Autodesk Inventor part; units mm, degrees
ref_plane "YZ Plane" through (0, 0, 0) normal (1, 0, 0) x (0, 1, 0)
ref_plane "XZ Plane" through (0, 0, 0) normal (0, 1, 0) x (-1, 0, 0)
ref_plane "XY Plane" through (0, 0, 0) normal (0, 0, 1) x (1, 0, 0)
sketch "Sketch1" plane through (0, 0, 0) normal (1, 0, 0) x (0, 1, 0)
  circle A0 centre (0, 0) radius 27.051
  dimension "d0" = 54.102
extrude "Extrusion1" add sketch "Sketch1" along normal blind 36.576
sketch "Sketch2" plane through (36.576, 0, 0) normal (1, 0, 0) x (0, 0, -1)
  circle A0 centre (0, 0) radius 6.35
  dimension "d3" = 12.7
extrude "Extrusion2" cut sketch "Sketch2" against normal through all
sketch "Sketch3" plane through (36.576, 0, 0) normal (1, 0, 0) x (0, 0, -1)
  circle A0 centre (0, 0) radius 6.35
  circle A1 centre (0, 0) radius 27.051
  line L0 (0, 0) -> (-36.068, 0) construction
  line L1 (-18.288, -6.0325) -> (-36.068, -6.0325)
  line L2 (-36.068, -6.0325) -> (-36.068, 6.0325)
  line L3 (-36.068, 6.0325) -> (-18.288, 6.0325)
  line L4 (-18.288, 6.0325) -> (-18.288, -6.0325)
  line L5 (-18.288, -6.0325) -> (-36.068, 6.0325) construction
  line L6 (-36.068, -6.0325) -> (-18.288, 6.0325) construction
  circle A2 centre (-30.734, 0) radius 2.921
  line L7 (-30.734, 2.921) -> (-36.068, 2.921)
  line L8 (-30.734, -2.921) -> (-36.068, -2.921)
  point P0 (-27.178, 0)
  dimension "d6" = 27.178
  dimension "d7" = 12.065
  dimension "d8" = 17.78
  dimension "d9" = 5.842
  dimension "d10" = 5.334
extrude "Extrusion3" add sketch "Sketch3" along normal blind 1.524 contours L3 L4 L1 A1 | A1 L1 L2 L8 A2 L7 L3 picked at (-21.1837, 0.6753)
properties part number "SlipRing"
Source: CAD feature listing. Evaluate the final solid. Frame: model axes, mm. A direction names the side the tool comes from. Coordinates: 2 decimals unless noted, no trailing zeros. Loops run counter-clockwise (first coordinate to the right, second up) from the corner with the lowest first, then second, coordinate; pieces in that order, holes last. Notation, with made-up numbers: (19, -11) - (75, -11) arc R7 cw to (75, -2) - close; hole circle Ø6 at (-35, -18). An arc over 180 degrees is marked (long way). One line per question, with ' | ' between items.
1) Pull-direction query (Y, two-part tool) for faces 4 (the face through (37, 2.921, 33)), 5 (the face through (37, -6.032, 27)), 6 (the face through (37, 6.032, 27)), 7 (the face through (18.54, -6.2, 1.38)); classes: released by +Y, released by -Y, zero draft, split by the parting line, or undercut.
Report:
face 4: undercut | face 5: released by -Y | face 6: released by +Y | face 7: undercut
2) Section C-C, the plane x = 21.5. Return loops of the section in (y, z).
Report:
outline: circle Ø54.1 at (0, 0); hole circle Ø12.7 at (0, 0)
3) First-contact query: P1, Ø2, axis at x = 27.5, z = 9, coming from the +Y side; P2, Ø1.5, axis at x = 10, z = 6, coming from the -Y side; P3, Ø10.5, axis at y = 0, z = 33.5, coming from the -X side. Flat tips, straight axial feed; report the tip coordinate or a pass-through.
Report:
P1: stops at y = 25.84 | P2: stops at y = -26.54 | P3: stops at x = 36.58
4) Set-up query: faces 1 (the face through (38.1, 0, 25)), 2 (the face through (37, -2.921, 33)), 3 (the face through (37, 0, 18.288)). Return all of +Z, -Z, +X, -X, +Y, -Y with unobstructed straight access to the full face (end or side cutting, diameter ignored); none if empty.
Report:
face 1: +Z, -Z, +X, +Y, -Y | face 2: +Z, +X, -X | face 3: -Z, +X, +Y, -Y
5) Section B-B, the plane z = 0. Return loops of the section in (x, y), then the cut area to 3 significant figures.
Report:
outline: (0, -27.05) - (36.58, -27.05) - (36.58, -6.35) - (0, -6.35) - close; (0, 6.35) - (36.58, 6.35) - (36.58, 27.05) - (0, 27.05) - close | area: 1,510 mm²
6) Section D-D, the plane y = 10. Return loops of the section in (x, z), then the cut area to 3 significant figures.
Report:
outline: (0, -25.13) - (36.58, -25.13) - (36.58, 25.13) - (0, 25.13) - close | area: 1,840 mm²
7) Line query: line 1 along Y through (x, z) = (27, 0); line 2 along X through (y, z) = (-15.5, 12.5); line 3 along Y through (x, z) = (6.5, -4). Output: solid intervals per line, ascending.
Report:
line 1: y = -27.05 to -6.35, 6.35 to 27.05 | line 2: x = 0 to 36.58 | line 3: y = -26.75 to -4.93, 4.93 to 26.75
8) Section A-A, the plane y = 0. Return loops of the section in (x, z), then the cut area to 3 significant figures.
Report:
outline: (0, -27.05) - (36.58, -27.05) - (36.58, -6.35) - (0, -6.35) - close; (0, 6.35) - (36.58, 6.35) - (36.58, 18.29) - (38.1, 18.29) - (38.1, 27.81) - (36.58, 27.81) - (36.58, 27.05) - (0, 27.05) - close | area: 1,530 mm²
